Work out the finished part from the listing and answer in its coordinate system (mm). A direction names the side the tool comes from. Give positions to 0.01 mm unless a question says otherwise; leave off trailing zeros. Loops run counter-clockwise (first coordinate to the right, second up) from the corner with the lowest first, then second, coordinate; pieces in that order, holes last. Notation, with made-up numbers: M -21,38.25 L 12,38.25 A15 ccw 12,47.25 Z; hole C 44.25,19 d1. An arc over 180 degrees is marked long. Write item = value, one per line. Start each with the question number.
1. Consider L1, parallel to Z at x = 5.5, y = 118; L2, parallel to X at y = 133.5, z = 9.75; L3, parallel to X at y = 125, z = -3.25. Determine where each line is inside the solid, lowest interval first. Write a range as [from, to].
2. Section C-C on x = -16 is taken. Determine the outline of the cut face in (y, z).
3. For faces 5 (the face through (14, 115, -8)), 6 (the face through (8, 125, 11)), 7 (the face through (0, 97, 12)), 8 (the face through (14, 86, -6.938)), 9 (the face through (1, 58, -11)), determine the directions among +Z, -Z, +X, -X, +Y, -Y from which every point of the face is accessible in a straight line to the end or side of a thin tool.
4. Section B-B on x = -5.5 is taken. Determine the outline of the cut face in (y, z), plus the area to 3 significant figures.
5. Flat-ended cylindrical pins translate along their axes: pin 1 Ø1.2 at (x, y) = (14, 74) entering from +Z; pin 2 Ø13 at (y, z) = (114, 1.5) entering from +X; pin 3 Ø1 at (y, z) = (126.5, 11) entering from -X; pin 4 Ø0.8 at (y, z) = (88.5, -9) entering from -X. Find the tip coordinate at first contact, or state that the pin passes through.
6. Section A-A on x = 2.5 is taken. Determine the outline of the cut face in (y, z).
7. The mould has two halves that part along X. Classify faces 1 (the face through (1, 138, -11)), 2 (the face through (-15, 97, 0)), 3 (the face through (14.57, 97.44, -10.96)), 4 (the face through (-14.653, 97.44, -10.903)): released by +X, released by -X, zero draft, split by the parting line, or undercut.
```python
from build123d import *

# Parameters (mm, degrees)
BOSS_EXTRUDE4_DEPTH = 80
BOSS_EXTRUDE5_DEPTH = 57
CUT_EXTRUDE1_DEPTH  = 2


with BuildPart() as part:
    # Sketch8 → Boss-Extrude4 (new body)
    with BuildSketch(Plane(origin=(0, 58, 0), x_dir=(1, 0, 0), z_dir=(0, 1, 0))):
        with BuildLine():
            Line((-11.194828593, 12.000000011), (11.194828559, 12.000000011))
            ThreePointArc((11.194828559, 12.000000011), (14.611088941, 10.932460351), (16.811684841, 8.109721678))
            add(Edge.make_bspline(
                [(18.334712564, 1.1e-08), (18.327162677, 2.726130673), (17.819510816, 5.426517656), (16.811684841, 8.109721678)],
                knots=[0.502499344, 0.502499344, 0.502499344, 0.502499344, 0.837905074, 0.837905074, 0.837905074, 0.837905074], degree=3))
            add(Edge.make_bspline(
                [(18.334712564, 1.1e-08), (18.327162677, -2.72613065), (17.819510816, -5.426517634), (16.811684841, -8.109721656)],
                knots=[0.502499344, 0.502499344, 0.502499344, 0.502499344, 0.837905074, 0.837905074, 0.837905074, 0.837905074], degree=3))
            ThreePointArc((16.811684841, -8.109721656), (14.611088941, -10.932460328), (11.194828559, -11.999999989))
            Line((11.194828559, -11.999999989), (-11.194828593, -11.999999989))
            ThreePointArc((-11.194828593, -11.999999989), (-14.611088975, -10.932460328), (-16.811684874, -8.109721656))
            add(Edge.make_bspline(
                [(-18.334712598, 1.1e-08), (-18.327162711, -2.72613065), (-17.81951085, -5.426517634), (-16.811684874, -8.109721656)],
                knots=[0.502499344, 0.502499344, 0.502499344, 0.502499344, 0.837905074, 0.837905074, 0.837905074, 0.837905074], degree=3))
            add(Edge.make_bspline(
                [(-18.334712598, 1.1e-08), (-18.327162711, 2.726130673), (-17.81951085, 5.426517656), (-16.811684874, 8.109721678)],
                knots=[0.502499344, 0.502499344, 0.502499344, 0.502499344, 0.837905074, 0.837905074, 0.837905074, 0.837905074], degree=3))
            ThreePointArc((-16.811684874, 8.109721678), (-14.611088975, 10.932460351), (-11.194828593, 12.000000011))
        make_face()
        with BuildLine():
            Line((-15.000000017, -7.999999989), (-15.000000017, 8.000000011))
            ThreePointArc((-15.000000017, 8.000000011), (-14.414213579, 9.414213574), (-13.000000017, 10.000000011))
            Line((-13.000000017, 10.000000011), (12.999999983, 10.000000011))
            ThreePointArc((12.999999983, 10.000000011), (14.414213546, 9.414213574), (14.999999983, 8.000000011))
            Line((14.999999983, 8.000000011), (14.999999983, -7.999999989))
            ThreePointArc((14.999999983, -7.999999989), (14.414213546, -9.414213551), (12.999999983, -9.999999989))
            Line((12.999999983, -9.999999989), (-13.000000017, -9.999999989))
            ThreePointArc((-13.000000017, -9.999999989), (-14.414213579, -9.414213551), (-15.000000017, -7.999999989))
        make_face(mode=Mode.SUBTRACT)
    extrude(amount=BOSS_EXTRUDE4_DEPTH)

    # Sketch11 → Boss-Extrude5 (add)
    with BuildSketch(Plane(origin=(0, 58, 0), x_dir=(1, 0, 0), z_dir=(0, 1, 0))):
        with BuildLine():
            Line((13, 10.000000011), (15, 10.000000011))
            Line((15, 10.000000011), (15, 6.937911183))
            Line((15, 6.937911183), (13.5, 6.937911183))
            ThreePointArc((13.5, 6.937911183), (13.146446609, 7.084357793), (13, 7.437911183))
            Line((13, 7.437911183), (13, 10.000000011))
        make_face()
        with BuildLine():
            Line((-13, 7.437911183), (-13, 10.000000011))
            Line((-13, 10.000000011), (-15, 10.000000011))
            Line((-15, 10.000000011), (-15, 6.937911183))
            Line((-15, 6.937911183), (-13.5, 6.937911183))
            ThreePointArc((-13.5, 6.937911183), (-13.146446609, 7.084357793), (-13, 7.437911183))
        make_face()
    extrude(amount=BOSS_EXTRUDE5_DEPTH)

    # Sketch12 → Cut-Extrude1 (cut)
    with BuildSketch(Plane.XY.offset(11.999999989)):
        with BuildLine():
            Line((7.5, 133.134156445), (7.5, 116.134156445))
            ThreePointArc((7.5, 116.134156445), (0, 108.634156445), (-7.5, 116.134156445))
            Line((-7.5, 116.134156445), (-7.5, 133.134156445))
            ThreePointArc((-7.5, 133.134156445), (-7.75, 133.384156445), (-8, 133.134156445))
            Line((-8, 133.134156445), (-8, 116.134156445))
            ThreePointArc((-8, 116.134156445), (0, 108.134156445), (8, 116.134156445))
            Line((8, 116.134156445), (8, 133.134156445))
            ThreePointArc((8, 133.134156445), (7.75, 133.384156445), (7.5, 133.134156445))
        make_face()
    extrude(amount=-CUT_EXTRUDE1_DEPTH, mode=Mode.SUBTRACT)


solid = part.part
```
Verdict:
q1.L1 = [-12, -10], [10, 12]
q1.L2 = [-15.88, -13.97], [13.97, 15.88]
q1.L3 = [-18.09, -15], [15, 18.09]
q2.outline = M 58,-9.59 L 138,-9.59 L 138,9.59 L 58,9.59 Z
q3.face_5 = +Y
q3.face_6 = +Z
q3.face_7 = +Z, +X, -X, +Y, -Y
q3.face_8 = +Y, -Y
q3.face_9 = +Z, -Z, +X, -X, -Y
q4.outline = M 58,-12 L 138,-12 L 138,-10 L 58,-10 Z; M 58,10 L 110.32,10 L 110.32,12 L 58,12 Z; M 111.04,10 L 138,10 L 138,12 L 111.04,12 Z
q4.area = 319 mm2
q5.pin_1 = 11.58
q5.pin_2 = 18.33
q5.pin_3 = -15.16
q5.pin_4 = -16.6
q6.outline = M 58,-12 L 138,-12 L 138,-10 L 58,-10 Z; M 58,10 L 108.53,10 L 108.53,12 L 58,12 Z; M 109.06,10 L 138,10 L 138,12 L 109.06,12 Z
q7.face_1 = zero draft
q7.face_2 = undercut
q7.face_3 = released by +X
q7.face_4 = released by -X
